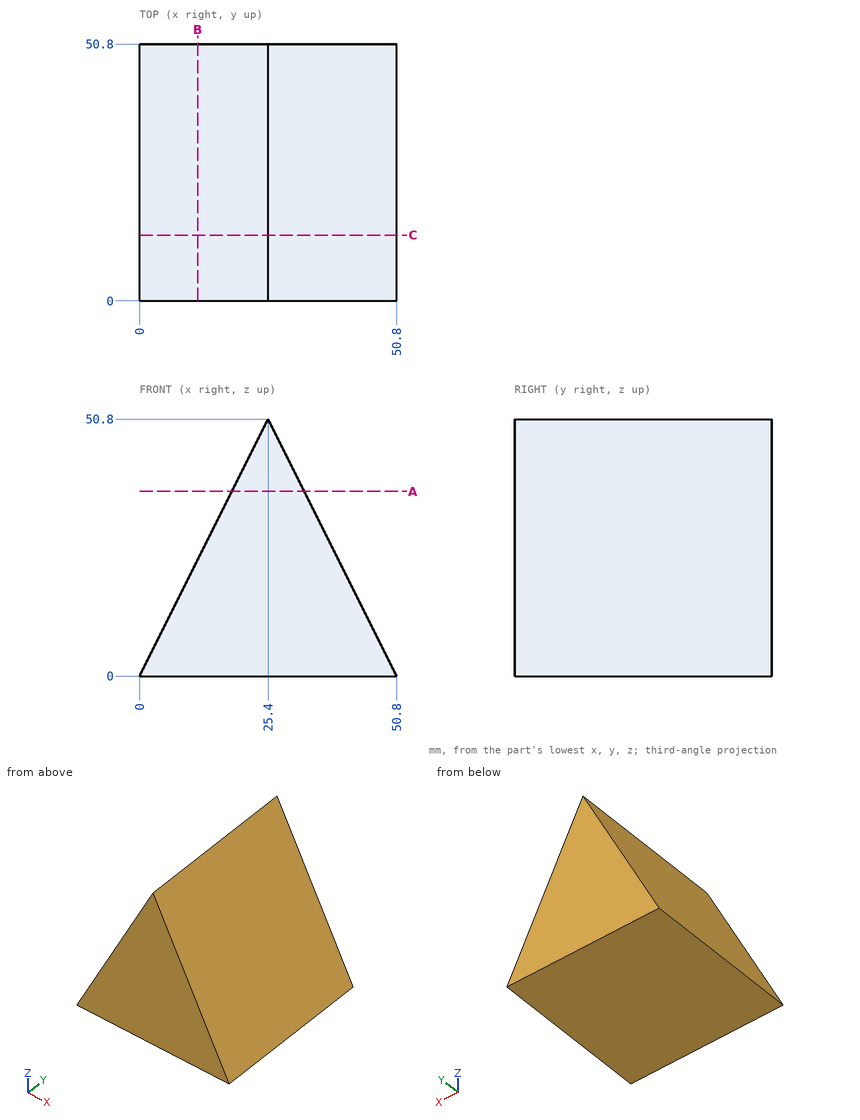
Can you work these out from the drawing? Everything is in mm from the part's minimum corner. Coordinates: 2 decimals unless noted, no trailing zeros. Loops run counter-clockwise (first coordinate to the right, second up) from the corner with the lowest first, then second, coordinate; pieces in that order, holes last.
1) Please list where these lines run through material, in increasing order: line 1 along Z through (x, y) = (37.5, 43.5); line 2 along X through (y, z) = (12, 27); line 3 along Z through (x, y) = (40, 47).
Reported:
line 1: z = 0 to 26.6
line 2: x = 13.5 to 37.3
line 3: z = 0 to 21.6
2) Imagine slicing it at A-A (z = 36.5). List the corners of the cut face in (x, y) for me.
Reported:
outline: (18.25, 0) - (32.55, 0) - (32.55, 50.8) - (18.25, 50.8) - close
3) Will these pins go through, and if not, where does the flat tip stop? pin 1 Ø1.5 at (y, z) = (21.5, 8.5) entering from +X (3 decimals); pin 2 Ø6 at (y, z) = (37.5, 22) entering from -X; pin 3 Ø6 at (y, z) = (16.5, 6.5) entering from -X.
Reported:
pin 1: stops at x = 46.925
pin 2: stops at x = 9.5
pin 3: stops at x = 1.75
4) Imagine slicing it at C-C (y = 13). List the corners of the cut face in (x, z) for me.
Reported:
outline: (0, 0) - (50.8, 0) - (25.4, 50.8) - close
5) Imagine slicing it at B-B (x = 11.5). List the corners of the cut face in (y, z) for me, and give its area (3 significant figures).
Reported:
outline: (0, 0) - (50.8, 0) - (50.8, 23) - (0, 23) - close
area: 1,170 mm2
